Could you check a few things on this model? Use its own coordinates, in mm. A direction names the side the tool comes from. Give positions to 0.01 mm unless a question says otherwise; leave off trailing zeros. Order: outer loops, then holes, each group sorted by start corner. A loop starts at its lowest first (then second) coordinate and runs counter-clockwise, first axis right, second up. Notation, with made-up numbers: M 79,14.5 L 120,14.5 A9 ccw 120,23.5 Z; hole C -9,37 d2. An arc over 180 degrees is marked long. Use a Markdown table: item, result. Add a question column.
Item 1: If we mould it in two halves opening along Z, with no side actions, what happens to faces 6 (the face through (-13, -24, 2)), 7 (the face through (0, 12.5, 4)), 8 (the face through (0, 0, 12)), 9 (the face through (-0.21, -11.64, 8.1))? For each: released by +Z, released by -Z, zero draft, split by the parting line, or undercut.
Item 2: Suppose I cut it at B-B on x = 0. Count the separate pieces of the cut face and the enclosed holes in it, plus the area to 3 significant figures.
Item 3: If I drill on L1, parallel to Y at x = 0, z = 1; L2, parallel to Y at x = 0, z = 4.65; L3, parallel to Z at x = -7.5, y = -1.5, over which ranges is the centre line in solid material (lowest first)? Write a range as from..to.
Item 4: Suppose I cut it at D-D on z = 1.5. Write out the boundary of the cut face in (x, y).
Item 5: Suppose I cut it at A-A on y = 0.5. Write out the boundary of the cut face in (x, z), plus the area to 3 significant figures.
Item 6: For faces 1 (the face through (0, -12.5, 4)), 2 (the face through (-0.2, 16.7, 5)), 3 (the face through (-0.12, -17.11, 3.99)), 4 (the face through (15, 0, 2)), 5 (the face through (0, -15, 7)), which set-ups out of +Z, -Z, +X, -X, +Y, -Y let a thin tool reach every point of the face, with its end or its side?
Item 7: I'm going to push flat-ended pins straight in: pin 1 Ø4 at (x, y) = (6, -19) entering from +Z; pin 2 Ø3 at (x, y) = (0, -19.856) entering from +Z; pin 3 Ø2 at (x, y) = (-2, 15) entering from +Z; pin 4 Ø7 at (x, y) = (0, 19.856) entering from -Z. Where does each tip first touch, or does it pass through?
Item 8: Suppose I cut it at C-C on x = -3.25. Write out the boundary of the cut face in (y, z).
Autodesk Fusion 360 part; units mm, degrees
sketch "Esquisse1" plane through (0, 0, 0) normal (0, 0, 1) x (1, 0, 0)
  line L0 (10, 25) -> (-10, 25)
  line L1 (-15, 20) -> (-15, -20)
  line L2 (-10, -25) -> (10, -25)
  line L3 (15, -20) -> (15, 20)
  line L4 (15, 25) -> (-15, -25) construction
  line L5 (-15, 25) -> (15, -25) construction
  line L6 (0, 0) -> (0, 40)
  line L7 (0, 40) -> (0, -29.6677)
  circle A0 centre (0, 20) radius 2.5
  circle A1 centre (0, -20) radius 2.5
  arc A2 (-10, 25) -> (-15, 20) centre (-10, 20) ccw
  arc A3 (15, 20) -> (10, 25) centre (10, 20) ccw
  arc A4 (10, -25) -> (15, -20) centre (10, -20) ccw
  arc A5 (-15, -20) -> (-10, -25) centre (-10, -20) ccw
  line L8 (-15, -15) -> (15, -15)
  line L9 (15, -15) -> (15, 15)
  line L10 (15, 15) -> (-15, 15)
  line L11 (-15, 15) -> (-15, -15)
  line L12 (-15, -15) -> (15, 15) construction
  line L13 (15, -15) -> (-15, 15) construction
  line L14 (-15, -12.5) -> (15, -12.5)
  line L15 (15, -12.5) -> (15, 12.5)
  line L16 (15, 12.5) -> (-15, 12.5)
  line L17 (-15, 12.5) -> (-15, -12.5)
  line L18 (-15, -12.5) -> (15, 12.5) construction
  line L19 (15, -12.5) -> (-15, 12.5) construction
  dimension "d1" = 30
  dimension "d2" = 50
  dimension "d3" = 5
  dimension "d4" = 5
  dimension "d5" = 5
  dimension "d6" = 5
  dimension "d7" = 5
  dimension "d8" = 5
  dimension "d9" = 30
  dimension "d10" = 30
  dimension "d20" = 25
extrude "Extrusion1" add sketch "Esquisse1" along normal blind 5 contours L0 L3 L6 L7 A0 A3 L10 | L0 L1 L6 L7 A0 A2 L10 | L2 L3 L7 A1 A4 L8 | L1 L2 L7 A1 A5 L8 makes body 1 at (-9.1574, 21.5425, 0) makes body 2 at (9.1574, -21.5425, 0)
extrude "Extrusion2" add sketch "Esquisse1" along normal blind 12 contours L3 L6 L7 L9 L10 L16 | L3 L6 L7 L9 L14 L15 L16 | L1 L6 L7 L10 L11 L16 | L3 L7 L8 L9 L14 | L1 L6 L7 L11 L14 L16 L17 | L1 L7 L8 L11 L14 bodies 1 2
extrude "Extrusion3" cut sketch "Esquisse1" along normal blind 9 contours L3 L6 L7 L9 L14 L15 L16 | L1 L6 L7 L11 L14 L16 L17 bodies 1
fillet "Congé1" radius 3 2 edges at (0, 15, 12) (0, -15, 12) on bodies 1
delete_face "DeleteFace1" 1 faces at (2.4876, -20.2489, 1.6667) on bodies 1
delete_face "DeleteFace2" 1 faces at (2.4876, 20.2489, 3.3333) on bodies 1
hole "Perçage1" at (0, 19.856, 5) direction (0, 0, -1) diameter 5 depth 5 tip angle 180 counterbore diameter 5.5 counterbore depth 2 bodies 1
hole "Perçage2" at (0, -19.856, 5) direction (0, 0, -1) diameter 5 depth 5 tip angle 180 counterbore diameter 5.5 counterbore depth 2 bodies 1
extrude "Extrusion4" add sketch "Esquisse1" along normal blind 3 contours L3 L6 L7 L9 L14 L15 L16 | L1 L6 L7 L11 L14 L16 L17 bodies 1
fillet "Congé2" radius 3 2 edges at (0, -12.5, 9) (0, 12.5, 9) on bodies 1
Findings below:
| question | item | result |
|---|---|---|
| 1 | face 6 | zero draft |
| 1 | face 7 | undercut |
| 1 | face 8 | released by +Z |
| 1 | face 9 | undercut |
| 2 | separate pieces | 3 |
| 2 | enclosed holes | 1 |
| 2 | area | 258 mm^2 |
| 3 | L1 | y = -25..-22.36, -17.36..17.36, 22.36..25 |
| 3 | L2 | y = -25..-22.61, -17.11..-12.5, 12.5..17.11, 22.61..25 |
| 3 | L3 | z = 0..3, 9..12 |
| 4 | outline | M -15,-20 A5 ccw -10,-25 L 10,-25 A5 ccw 15,-20 L 15,20 A5 ccw 10,25 L -10,25 A5 ccw -15,20 Z; hole C 0,-19.86 d5; hole C 0,19.86 d5 |
| 5 | outline | M -15,0 L 15,0 L 15,3 L -15,3 Z; M -15,9 L 15,9 L 15,12 L -15,12 Z |
| 5 | area | 180 mm^2 |
| 6 | face 1 | +X, -X |
| 6 | face 2 | +Z, +X, -X, +Y |
| 6 | face 3 | +Z |
| 6 | face 4 | +Z, -Z, +X, +Y, -Y |
| 6 | face 5 | +Z, +X, -X, -Y |
| 7 | pin 1 | stops at z = 5 |
| 7 | pin 2 | passes through |
| 7 | pin 3 | stops at z = 11.24 |
| 7 | pin 4 | stops at z = 0 |
| 8 | outline | M -25,0 L 25,0 L 25,5 L 15,5 L 15,9 A3 ccw 12,12 L -12,12 A3 ccw -15,9 L -15,5 L -25,5 Z; hole M -12.5,3 L 12.5,3 L 12.5,6 A3 ccw 9.5,9 L -9.5,9 A3 ccw -12.5,6 Z |
